Read the model definition and answer for the solid it produces. Units are mm, in the model's axes. A direction names the side the tool comes from. Give positions to 0.01 mm unless a question says otherwise; leave off trailing zeros. Write each loop counter-clockwise with the first axis right and the second up, starting at its lowest first coordinate (ties: lowest second). Pieces come first, ordered by that corner, then holes. Notation, with made-up numbers: M -23.5,47.25 L 21.5,47.25 A22 ccw 21.5,86.25 Z; hole C 71.25,60.5 d1. An arc over 180 degrees is marked long. Write each question's results on one line, items separated by ' | '. Start each with the question number.
```python
from build123d import *

# Parameters (mm, degrees)
SALIENTE_EXTRUIR1_DEPTH = 25
CROQUIS2_W              = 72.044924806
CROQUIS2_H              = 8
SALIENTE_EXTRUIR2_DEPTH = 50
CROQUIS3_R              = 10
CORTAR_EXTRUIR1_DEPTH   = 50


with BuildPart() as part:
    # Croquis1 → Saliente-Extruir1 (new, symmetric)
    with BuildSketch(Plane.XY):
        with BuildLine():
            Line((0, 0), (50, 0))
            Line((50, 0), (50, 50))
            ThreePointArc((50, 50), (47.5, 52.5), (45, 50))
            Line((45, 50), (45, 15))
            ThreePointArc((45, 15), (42.071067812, 7.928932188), (35, 5))
            Line((35, 5), (0, 5))
            ThreePointArc((0, 5), (-2.5, 2.5), (0, 0))
        make_face()
    extrude(amount=SALIENTE_EXTRUIR1_DEPTH, both=True)

    # Croquis2 → Saliente-Extruir2 (add)
    with BuildSketch(Plane.XZ):
        with Locations((13.977537597, 0.439965546)):
            Rectangle(CROQUIS2_W, CROQUIS2_H)
    extrude(amount=SALIENTE_EXTRUIR2_DEPTH)

    # Croquis3 → Cortar-Extruir1 (cut)
    with BuildSketch(Plane.XY.offset(4.439965546)):
        with Locations((0, -25.510653739)):
            Circle(CROQUIS3_R)
    extrude(amount=-CORTAR_EXTRUIR1_DEPTH, mode=Mode.SUBTRACT)


solid = part.part
```
Item 1: Section B-B, the plane x = 47.5 is taken. Determine the outline of the cut face in (y, z), then the cut area to 4 significant figures.
Item 2: Given P1, Ø10.5, axis at y = 26, z = -5.5, coming from the -X side; P2, Ø25, axis at x = 16, y = -29.5, coming from the +Z side; P3, Ø9, axis at x = -5.5, z = 1, coming from the +Y side, each flat-ended and moving along its own axis, determine where each tip first touches the part or whether it passes through.
Item 3: Determine the mould class of faces 5 (the cylindrical face through (47.6, 52.5, 0.4)), 6 (the flat face through (-22.045, -25, 0)), 7 (the flat face through (37, 5, -25)), 8 (the cylindrical face through (5.38, -17.08, 0.5)) for opening direction X: +X half, -X half, draft (parallel to the pull), parting line (faces both ways), or undercut.
Item 4: Section A-A, the plane x = -6 is taken. Determine the outline of the cut face in (y, z), then the cut area to 3 significant figures.
Item 5: Straight lines are drawn through the part: line 1 (X direction, y = 15, z = 1); line 2 (Z direction, x = 13, y = -18); line 3 (Y direction, x = 27.5, z = 13.5). For each, find the intervals that lie inside material, in ascending order.
Item 6: Section D-D, the plane y = 2.5 is taken. Determine the outline of the cut face in (x, z).
Item 7: For faces 1 (the flat face through (45, 33, 0)), 2 (the flat face through (50, 23, 0)), 3 (the flat face through (25, 0, 15)), 4 (the flat face through (13, -25, -3.56)), determine the directions among +Z, -Z, +X, -X, +Y, -Y from which every point of the face is accessible in a straight line to the end or side of a thin tool.
Item 8: Section C-C, the plane z = 10 is taken. Determine the outline of the cut face in (x, y).
Worked out:
1) outline: M -50,-3.56 L 0,-3.56 L 0,-25 L 52.5,-25 L 52.5,25 L 0,25 L 0,4.44 L -50,4.44 Z | area: 3,025 mm²
2) P1: stops at x = 45 | P2: stops at z = 4.44 | P3: stops at y = 4.79
3) face 5: parting line | face 6: -X half | face 7: draft | face 8: undercut
4) outline: M -50,-3.56 L -33.51,-3.56 L -33.51,4.44 L -50,4.44 Z; M -17.51,-3.56 L 0,-3.56 L 0,4.44 L -17.51,4.44 Z | area: 272 mm²
5) line 1: x = 45 to 50 | line 2: z = -3.56 to 4.44 | line 3: y = 0 to 5
6) outline: M -2.5,-25 L 50,-25 L 50,25 L -2.5,25 Z
7) face 1: +Z, -Z, -X, +Y | face 2: +Z, -Z, +X, +Y, -Y | face 3: +Z, +X, -X, -Y | face 4: -Z, +X, -X, -Y
8) outline: M 0,0 L 50,0 L 50,50 A2.5 ccw 45,50 L 45,15 A10 cw 35,5 L 0,5 A2.5 ccw Z
